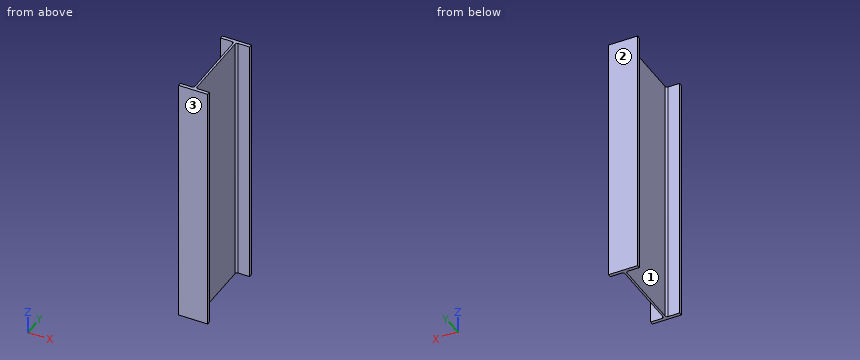
Autodesk Inventor part; units mm, degrees
ref_plane "Start plane" through (0, 0, 0) normal (0, 0, 1) x (1, 0, 0)
ref_plane "End plane" through (0, 0, 2375) normal (0, 0, 1) x (1, 0, 0)
ref_plane "YZ Plane" through (0, 0, 0) normal (1, 0, 0) x (0, 1, 0)
ref_plane "Start plane" through (0, 0, 0) normal (0, 0, 1) x (1, 0, 0)
ref_plane "End plane" through (0, 0, 2375) normal (0, 0, 1) x (1, 0, 0)
sketch "Sketch" plane through (0, 0, 0) normal (0, 0, 1) x (1, 0, 0)
  line L0 (-136, -390.5) -> (-136, -359.2)
  line L1 (-136, -359.2) -> (-26.15, -359.2)
  line L2 (-9.65, -342.7) -> (-9.65, 0)
  line L3 (-9.65, 0) -> (0, 0) construction
  line L4 (0, 0) -> (0, -390.5) construction
  line L5 (0, -390.5) -> (-136, -390.5)
  line L6 (-60, 0) -> (80, 0) construction
  line L7 (0, -60) -> (0, 80) construction
  line L8 (136, -390.5) -> (136, -359.2)
  line L9 (136, -359.2) -> (26.15, -359.2)
  line L10 (9.65, -342.7) -> (9.65, 0)
  line L11 (9.65, 0) -> (0, 0) construction
  line L12 (0, -390.5) -> (136, -390.5)
  line L13 (-136, 390.5) -> (-136, 359.2)
  line L14 (-136, 359.2) -> (-26.15, 359.2)
  line L15 (-9.65, 342.7) -> (-9.65, 0)
  line L16 (0, 390.5) -> (-136, 390.5)
  line L17 (136, 390.5) -> (136, 359.2)
  line L18 (136, 359.2) -> (26.15, 359.2)
  line L19 (0, 390.5) -> (136, 390.5)
  line L20 (9.65, 342.7) -> (9.65, 0)
  arc A0 (-9.65, 342.7) -> (-26.15, 359.2) centre (-26.15, 342.7) ccw
  arc A1 (26.15, 359.2) -> (9.65, 342.7) centre (26.15, 342.7) ccw
  arc A2 (9.65, -342.7) -> (26.15, -359.2) centre (26.15, -342.7) ccw
  arc A3 (-26.15, -359.2) -> (-9.65, -342.7) centre (-26.15, -342.7) ccw
  line L21 (0, 108) -> (0, -88) construction
  line L22 (-88, 0) -> (108, 0) construction
  point P0 (-9.65, -359.2)
  point P1 (9.65, -359.2)
  point P2 (-9.65, 359.2)
  point P3 (9.65, 359.2)
  dimension "d1" = 390.5
  dimension "d2" = 31.3
  dimension "d3" = 136
  dimension "d4" = 9.65
  dimension "d10" = 16.5
extrude "Body" add sketch "Sketch" along normal up to surface (2375 mm away) from surface at 0
sketch "Sketch4" plane through (0, 0, 0) normal (0, 0, 1) x (1, 0, 0)
  line L0 (0, 0) -> (10, 0)
ref_plane "Work Plane3" through (0, 0, 0) normal (0, -1, 0) x (1, 0, 0)
sketch "Sketch5" plane through (0, 0, 0) normal (0, -1, 0) x (1, 0, 0)
  line L0 (-2, 0) -> (12, 0)
  line L1 (-2, 2375) -> (12, 2375)
  dimension "d14" = 2375
equation "\"d1\" = 0.5 * G_H"
equation "\"d2\" = G_T1"
equation "\"d3\" = 0.5 * G_W"
equation "\"d4\" = 0.5 * G_T"
equation "\"d10\" = G_IR"
equation "\"d5\" = G_L"
equation "\"G_W\" = 272"
equation "\"G_H\" = 781"
equation "\"G_T\" = 19.3"
equation "\"G_T1\" = 31.3"
equation "\"G_IR\" = 16.5"
equation "\"G_L\" = d14"
equation "\"G_OFFSET_START\" = 0"
equation "\"G_OFFSET_END\" = 0"
equation "\"d12\" = G_OFFSET_END + B_L"
equation "\"B_L\" = 2375"
properties part number "AS 3679-1990 - 760 UB - 244 - 2375" material "Steel, Mild"
Part model, mm, in its own coordinate system. Face numbers are marked on the shaded views. Coordinates: 2 decimals unless noted, no trailing zeros. Loops run counter-clockwise (first coordinate to the right, second up) from the corner with the lowest first, then second, coordinate; pieces in that order, holes last. Notation, with made-up numbers: M 56,49 L 63,49 A28 cw 63,72 Z; hole C 59,-40 d2. An arc over 180 degrees is marked long. Use a Markdown table: item, result. Add a question column.
Q1. Mould opens along Y. For the marked faces 1, 2 and 3 say: +Y half, -Y half, draft (parallel to the pull), parting line (faces both ways), or undercut.
Q2. Probe L1, parallel to Y at x = -87, z = 1980; L2, parallel to X at y = -10.5, z = 1221.5; L3, parallel to Y at x = -20, z = 1805. List the from-to ranges inside material, lowest first.
Q3. Cut at B-B (z = 1746.5). Write the cut outline in (x, y).
Q4. Pin check, flat tips, straight feed: P1, Ø4, axis at y = -146, z = 833.5, coming from the +X side; P2, Ø10, axis at y = -133.5, z = 759, coming from the -X side. Stop position of each tip, or through.
Q5. Cut at A-A (x = -60.5). Write the cut outline in (y, z).
Q6. Cut at C-C (y = -22). Write the cut outline in (x, z), and give its area (3 significant figures).
Worked out:
| question | item | result |
|---|---|---|
| 1 | face 1 | undercut |
| 1 | face 2 | +Y half |
| 1 | face 3 | -Y half |
| 2 | L1 | y = -390.5 to -359.2, 359.2 to 390.5 |
| 2 | L2 | x = -9.65 to 9.65 |
| 2 | L3 | y = -390.5 to -358.01, 358.01 to 390.5 |
| 3 | outline | M -136,-390.5 L 136,-390.5 L 136,-359.2 L 26.15,-359.2 A16.5 cw 9.65,-342.7 L 9.65,342.7 A16.5 cw 26.15,359.2 L 136,359.2 L 136,390.5 L -136,390.5 L -136,359.2 L -26.15,359.2 A16.5 cw -9.65,342.7 L -9.65,-342.7 A16.5 cw -26.15,-359.2 L -136,-359.2 Z |
| 4 | P1 | stops at x = 9.65 |
| 4 | P2 | stops at x = -9.65 |
| 5 | outline | M -390.5,0 L -359.2,0 L -359.2,2375 L -390.5,2375 Z; M 359.2,0 L 390.5,0 L 390.5,2375 L 359.2,2375 Z |
| 6 | outline | M -9.65,0 L 9.65,0 L 9.65,2375 L -9.65,2375 Z |
| 6 | area | 45,800 mm2 |
